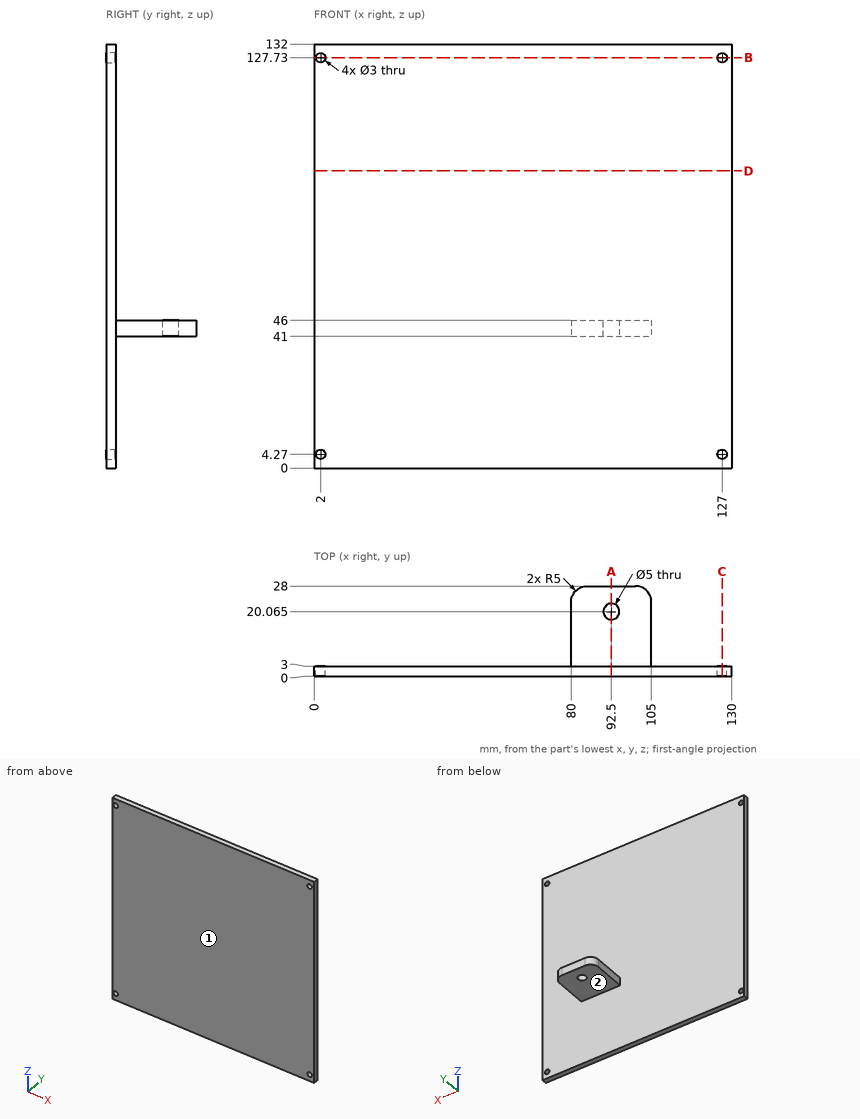
Geometry check sheet. Reference: drawing and pictorial views, mm from the part's lowest x, y, z. Coordinates: 2 decimals unless noted, no trailing zeros. Write each loop counter-clockwise with the first axis right and the second up, starting at its lowest first coordinate (ties: lowest second). Pieces come first, ordered by that corner, then holes.
Item 1: Cross-section at B-B on z = 127.73. Record the boundary of the cut face in (x, y), then the cut area to 3 significant figures.
Numbers:
outline: (0, 0) - (0.5, 0) - (0.5, 3) - (0, 3) - close; (3.5, 0) - (125.5, 0) - (125.5, 3) - (3.5, 3) - close; (128.5, 0) - (130, 0) - (130, 3) - (128.5, 3) - close
area: 372 mm2
Item 2: Mould release check, pull along Z, two halves, no side actions. Record for the marked faces 1 and 2: released by +Z, released by -Z, zero draft, split by the parting line, or undercut.
Numbers:
face 1: zero draft
face 2: released by -Z
Item 3: Cross-section at A-A on x = 92.5. Record the boundary of the cut face in (y, z) (1 decimal), then the cut area to 3 significant figures.
Numbers:
outline: (0, 0) - (3, 0) - (3, 41) - (17.6, 41) - (17.6, 46) - (3, 46) - (3, 132) - (0, 132) - close; (22.6, 41) - (28, 41) - (28, 46) - (22.6, 46) - close
area: 496 mm2
Item 4: Depth check by flat-ended pin: pin 1 Ø8 at (x, y) = (100.5, 5.5) entering from +Z; pin 2 Ø2.5 at (y, z) = (9, 44) entering from -X; pin 3 Ø5.5 at (y, z) = (16.5, 43) entering from +X; pin 4 Ø3 at (x, y) = (98, 18) entering from +Z. Enter the tip coordinate at first touch or a pass-through.
Numbers:
pin 1: stops at z = 132
pin 2: stops at x = 80
pin 3: stops at x = 105
pin 4: stops at z = 46
Item 5: Scan lines: probe 1 along X at (y, z) = (1.95, 127.73); probe 2 along Z at (x, y) = (2, 0.7); probe 3 along Y at (x, z) = (96, 96). Record each from-to range of solid material in increasing order.
Numbers:
probe 1: x = 0 to 0.5, 3.5 to 125.5, 128.5 to 130
probe 2: z = 0 to 2.77, 5.77 to 126.23, 129.23 to 132
probe 3: y = 0 to 3
Item 6: Cross-section at D-D on z = 92.5. Record the boundary of the cut face in (x, y), then the cut area to 3 significant figures.
Numbers:
outline: (0, 0) - (130, 0) - (130, 3) - (0, 3) - close
area: 390 mm2
Item 7: Cross-section at C-C on x = 127. Record the boundary of the cut face in (y, z), then the cut area to 3 significant figures.
Numbers:
outline: (0, 0) - (3, 0) - (3, 2.77) - (0, 2.77) - close; (0, 5.77) - (3, 5.77) - (3, 126.23) - (0, 126.23) - close; (0, 129.23) - (3, 129.23) - (3, 132) - (0, 132) - close
area: 378 mm2
